Input: part model. Units: mm. Frame: model coordinates. Give positions to 0.01 mm unless a question says otherwise; leave off trailing zeros. Loops run counter-clockwise (first coordinate to the right, second up) from the corner with the lowest first, then second, coordinate; pieces in that order, holes last. Notation, with made-up numbers: (55.25, 43) -> (99.25, 43) arc R14 ccw to (99.25, 59) -> close; hole circle Ø7 at (-8, 61). An arc over 180 degrees is marked (long way). Answer as a JSON object with one key per item and string values.
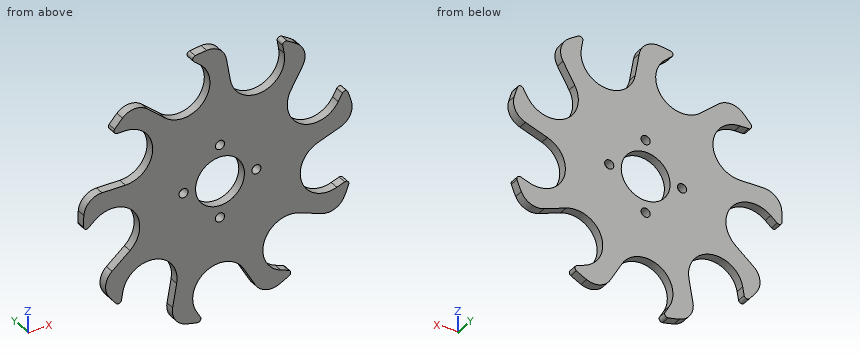
```python
from build123d import *

# Parameters (mm, degrees)
SKETCH_1_R      = 8.05
SKETCH_1_R_2    = 1.5
EXTRUDE_1_DEPTH = 3


with BuildPart() as part:
    # 草图1 → 凸台-拉伸1 (new body)
    with BuildSketch(Plane(origin=(0, 3, 0), x_dir=(1, 0, 0), z_dir=(0, 1, 0))):
        with BuildLine():
            Line((-38.88444419, -9), (-31.176914536, -9))
            ThreePointArc((-31.176914536, -9), (-22.176914536, -18), (-31.176914536, -27))
            Line((-31.176914536, -27), (-33.941125497, -27))
            ThreePointArc((-33.941125497, -27), (-34.845659531, -27.573598567), (-34.712514713, -28.636363636))
            ThreePointArc((-34.712514713, -28.636363636), (-33.459137261, -30.091296644), (-32.144826423, -31.491429536))
            ThreePointArc((-32.144826423, -31.491429536), (-28.151334956, -33.285439049), (-24.002123909, -31.888838923))
            Line((-24.002123909, -31.888838923), (-18.097813647, -26.93453436))
            ThreePointArc((-18.097813647, -26.93453436), (-5.418325172, -28.043845861), (-6.527636673, -40.723334336))
            Line((-6.527636673, -40.723334336), (-8.645145119, -42.500134892))
            ThreePointArc((-8.645145119, -42.500134892), (-8.969356337, -43.520960157), (-8.18422927, -44.249501593))
            ThreePointArc((-8.18422927, -44.249501593), (-6.288873528, -44.558389443), (-4.382064939, -44.786130742))
            ThreePointArc((-4.382064939, -44.786130742), (-0.169705906, -43.593454926), (2.111056904, -39.856535709))
            Line((2.111056904, -39.856535709), (3.449455383, -32.266100749))
            ThreePointArc((3.449455383, -32.266100749), (13.875558759, -24.965664571), (21.175994937, -35.391767947))
            Line((21.175994937, -35.391767947), (20.695994741, -38.113984332))
            ThreePointArc((20.695994741, -38.113984332), (21.10380837, -39.104380808), (22.173548005, -39.157805976))
            ThreePointArc((22.173548005, -39.157805976), (23.824024022, -38.17611661), (25.431113431, -37.124903632))
            ThreePointArc((25.431113431, -37.124903632), (27.891330424, -33.503608756), (27.236450729, -29.174916481))
            Line((27.236450729, -29.174916481), (23.382685902, -22.5))
            ThreePointArc((23.382685902, -22.5), (26.676914536, -10.205771366), (38.97114317, -13.5))
            Line((38.97114317, -13.5), (40.353248651, -15.893876913))
            ThreePointArc((40.353248651, -15.893876913), (41.302266598, -16.390427082), (42.156075737, -15.743737752))
            ThreePointArc((42.156075737, -15.743737752), (42.789395957, -13.930814535), (43.344791191, -12.092521515))
            ThreePointArc((43.344791191, -12.092521515), (42.901703271, -7.737051698), (39.617606559, -4.842029588))
            Line((39.617606559, -4.842029588), (32.374897819, -2.205899191))
            ThreePointArc((32.374897819, -2.205899191), (26.995845521, 9.329515686), (38.531260398, 14.708567983))
            Line((38.531260398, 14.708567983), (41.12876904, 13.763152154))
            ThreePointArc((41.12876904, 13.763152154), (42.174935261, 13.992789635), (42.41330712, 15.037000338))
            ThreePointArc((42.41330712, 15.037000338), (41.733133973, 16.832870485), (40.97695943, 18.598085813))
            ThreePointArc((40.97695943, 18.598085813), (37.837892358, 21.649757837), (33.461243979, 21.756496762))
            Line((33.461243979, 21.756496762), (26.218535239, 19.120366365))
            ThreePointArc((26.218535239, 19.120366365), (14.683120362, 24.499418662), (20.062172659, 36.034833539))
            Line((20.062172659, 36.034833539), (22.659681301, 36.980249368))
            ThreePointArc((22.659681301, 36.980249368), (23.313482993, 37.828624569), (22.824880729, 38.781758852))
            ThreePointArc((22.824880729, 38.781758852), (21.149474791, 39.720268328), (19.435552943, 40.586442093))
            ThreePointArc((19.435552943, 40.586442093), (15.06931109, 40.906405071), (11.647993461, 38.174916481))
            Line((11.647993461, 38.174916481), (7.794228634, 31.5))
            ThreePointArc((7.794228634, 31.5), (-4.5, 28.205771366), (-7.794228634, 40.5))
            Line((-7.794228634, 40.5), (-6.412123154, 42.893876913))
            ThreePointArc((-6.412123154, 42.893876913), (-6.456607068, 43.964025649), (-7.443561025, 44.380101389))
            ThreePointArc((-7.443561025, 44.380101389), (-9.330258696, 44.022111179), (-11.199964768, 43.583951051))
            ThreePointArc((-11.199964768, 43.583951051), (-14.750368314, 41.022490747), (-15.61548265, 36.730868511))
            Line((-15.61548265, 36.730868511), (-14.277084172, 29.140433551))
            ThreePointArc((-14.277084172, 29.140433551), (-21.57752035, 18.714330175), (-32.003623726, 26.014766353))
            Line((-32.003623726, 26.014766353), (-32.483623922, 28.736982738))
            ThreePointArc((-32.483623922, 28.736982738), (-33.205578925, 29.528170522), (-34.229077849, 29.212501255))
            ThreePointArc((-34.229077849, 29.212501255), (-35.444260445, 27.725518958), (-36.59489449, 26.18804493))
            ThreePointArc((-36.59489449, 26.18804493), (-37.668186452, 21.943697089), (-35.572300883, 18.100038947))
            Line((-35.572300883, 18.100038947), (-29.667990621, 13.145734384))
            ThreePointArc((-29.667990621, 13.145734384), (-28.55867912, 0.466245909), (-41.238167596, -0.643065592))
            Line((-41.238167596, -0.643065592), (-43.355676042, 1.133734964))
            ThreePointArc((-43.355676042, 1.133734964), (-44.417291364, 1.275756238), (-44.998428734, 0.376047124))
            ThreePointArc((-44.998428734, 0.376047124), (-44.973498813, -1.544151718), (-44.866666374, -3.461538462))
            ThreePointArc((-44.866666374, -3.461538462), (-42.960641513, -7.402796314), (-38.88444419, -9))
        make_face()
        with Locations(Location((0, 0, 0), (0, 0, 90))):
            Circle(SKETCH_1_R, mode=Mode.SUBTRACT)
        with Locations(Location((0, 12, 0), (0, 0, 270))):
            Circle(SKETCH_1_R_2, mode=Mode.SUBTRACT)
        with Locations(Location((12, 0, 0), (0, 0, 270))):
            Circle(SKETCH_1_R_2, mode=Mode.SUBTRACT)
        with Locations(Location((0, -12, 0), (0, 0, 270))):
            Circle(SKETCH_1_R_2, mode=Mode.SUBTRACT)
        with Locations(Location((-12, 0, 0), (0, 0, 270))):
            Circle(SKETCH_1_R_2, mode=Mode.SUBTRACT)
    extrude(amount=-EXTRUDE_1_DEPTH)


solid = part.part
```
Q1. Ray query, line 1 along X through (y, z) = (1.65, 0); line 2 along X through (y, z) = (1.6, 31.5); line 3 along X through (y, z) = (0.4, -40.5). Return the intervals inside material, ascending.
Evaluation:
{"line 1": "x = -45 to -42, -28.98 to -13.5, -10.5 to -8.05, 8.05 to 10.5, 13.5 to 28.98", "line 2": "x = -32.14 to -23.54, -3.62 to 3.62, 21.01 to 28", "line 3": "x = -15.05 to -7.79, 14.08 to 19.62"}
Q2. Section A-A, the plane z = -3. Return the cut outline in (x, y).
Evaluation:
{"outline": "(-27.06, 0) -> (-7.47, 0) -> (-7.47, 3) -> (-27.06, 3) -> close; (7.47, 0) -> (27.06, 0) -> (27.06, 3) -> (7.47, 3) -> close"}
Q3. Section D-D, the plane x = 0. Return the cut outline in (y, z).
Evaluation:
{"outline": "(0, -27) -> (3, -27) -> (3, -13.5) -> (0, -13.5) -> close; (0, -10.5) -> (3, -10.5) -> (3, -8.05) -> (0, -8.05) -> close; (0, 8.05) -> (3, 8.05) -> (3, 10.5) -> (0, 10.5) -> close; (0, 13.5) -> (3, 13.5) -> (3, 43.46) -> (0, 43.46) -> close"}
Q4. Section C-C, the plane y = 0.9. Give the number of separate pieces and of enclosed holes in the cut face, then the cut area to 3 significant figures.
Evaluation:
{"separate pieces": "1", "enclosed holes": "5", "area": "3,360 mm2"}
Q5. Pin query (flat end, axial travel): pin 1 (1.5 mm diameter, centred on x = 19.5, y = 1.5, fed in from -Z). Return the tip coordinate at first contact, or that it passes through.
Evaluation:
{"pin 1": "stops at z = -40.86"}
Q6. Section B-B, the plane x = 17.5. Return the cut outline in (y, z).
Evaluation:
{"outline": "(0, -41.14) -> (3, -41.14) -> (3, -34.59) -> (0, -34.59) -> close; (0, -20.56) -> (3, -20.56) -> (3, 26.47) -> (0, 26.47) -> close"}
